Design review of the part shown in the three views and the two pictorial views. Dimensions are in mm from the part's minimum x, y and z. Round coordinates to 2 decimals unless told otherwise and drop trailing zeros. Loops run counter-clockwise (first coordinate to the right, second up) from the corner with the lowest first, then second, coordinate; pieces in that order, holes last. Notation, with made-up numbers: M 25,27.5 L 79,27.5 A32 ccw 79,60.5 Z; hole C 2.5,81 d4. An arc over 180 degrees is marked long. Return JSON: item names as keys, results as strings. Group by question number.
Q1. To check wall thickness, follow line 1 along X through (y, z) = (0.25, 9.75); line 2 along X through (y, z) = (1.05, 20); line 3 along Z through (x, y) = (6.25, 0.35). State the ranges of each line that lie inside material, in increasing order.
Q2. Clearance check with flat-ended pins moving along their axes: pin 1 Ø0.5 at (y, z) = (0.5, 13) entering from -X; pin 2 Ø0.8 at (y, z) = (0.5, 19.5) entering from -X. State where each tip first meets the part, or that it passes through.
Q3. Consider section C-C (x = 1.25). State the section outline as (y, z) points.
Q4. Consider section B-B (y = 1.2). State the section outline as (x, z) points, and give its area (3 significant figures).
Q5. Consider section D-D (z = 18.75). State the section outline as (x, y) points.
Q6. Consider section A-A (z = 12.75). State the section outline as (x, y) points, and give its area (3 significant figures).
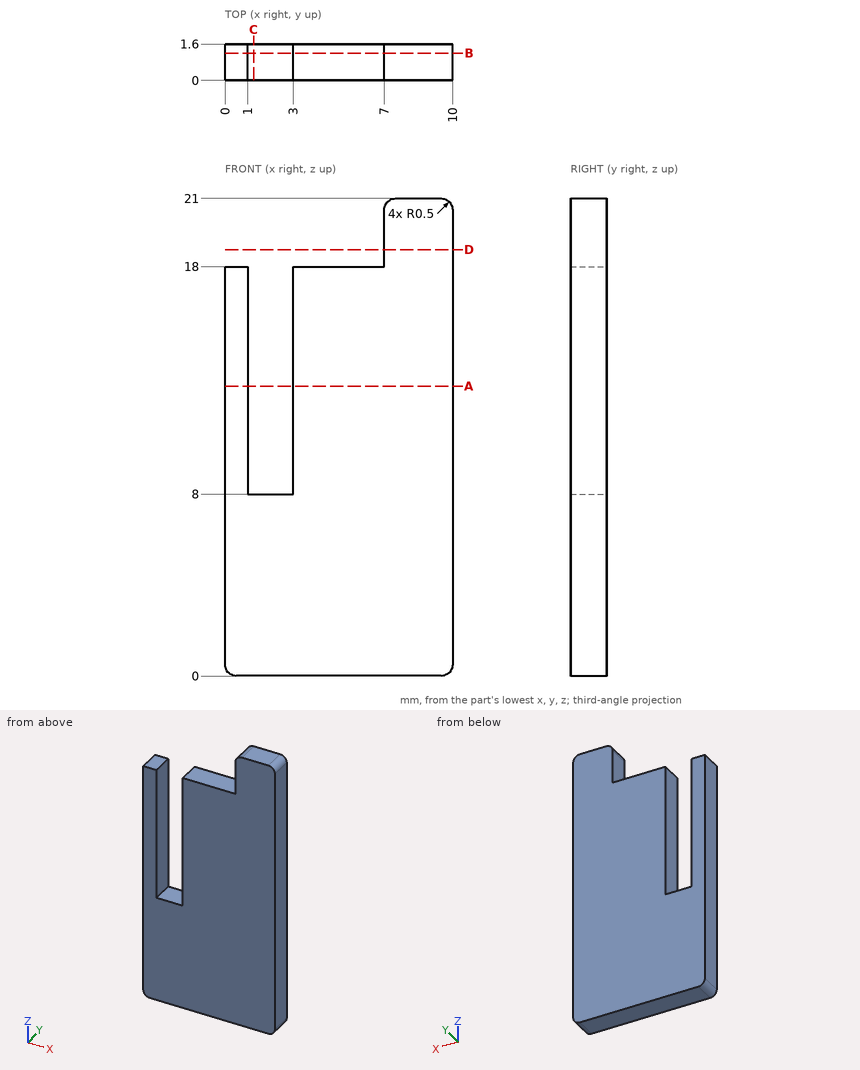
Values:
{
 "1": {"line 1": "x = 0 to 1, 3 to 10", "line 2": "x = 7 to 10", "line 3": "z = 0 to 18"},
 "2": {"pin 1": "stops at x = 0", "pin 2": "stops at x = 7"},
 "3": {"outline": "M 0,0 L 1.6,0 L 1.6,8 L 0,8 Z"},
 "4": {"outline": "M 0,0.5 A0.5 ccw 0.5,0 L 9.5,0 A0.5 ccw 10,0.5 L 10,20.5 A0.5 ccw 9.5,21 L 7.5,21 A0.5 ccw 7,20.5 L 7,18 L 3,18 L 3,8 L 1,8 L 1,18 L 0,18 Z", "area": "169 mm2"},
 "5": {"outline": "M 7,0 L 10,0 L 10,1.6 L 7,1.6 Z"},
 "6": {"outline": "M 0,0 L 1,0 L 1,1.6 L 0,1.6 Z; M 3,0 L 10,0 L 10,1.6 L 3,1.6 Z", "area": "12.8 mm2"}
}
